The drawing under review shows one solid part. Ordinate dimensions are in mm from its lowest x, y, z. A direction names the side the tool comes from. Coordinates: 2 decimals unless noted, no trailing zeros. Loops run counter-clockwise (first coordinate to the right, second up) from the corner with the lowest first, then second, coordinate; pieces in that order, holes last. Notation, with made-up numbers: M 28,38 L 80,38 A22 cw 80,75 Z; hole C 65.25,41.25 d7. An arc over 180 degrees is marked long. Answer as CSV lines item,"result". Start each with the question number.
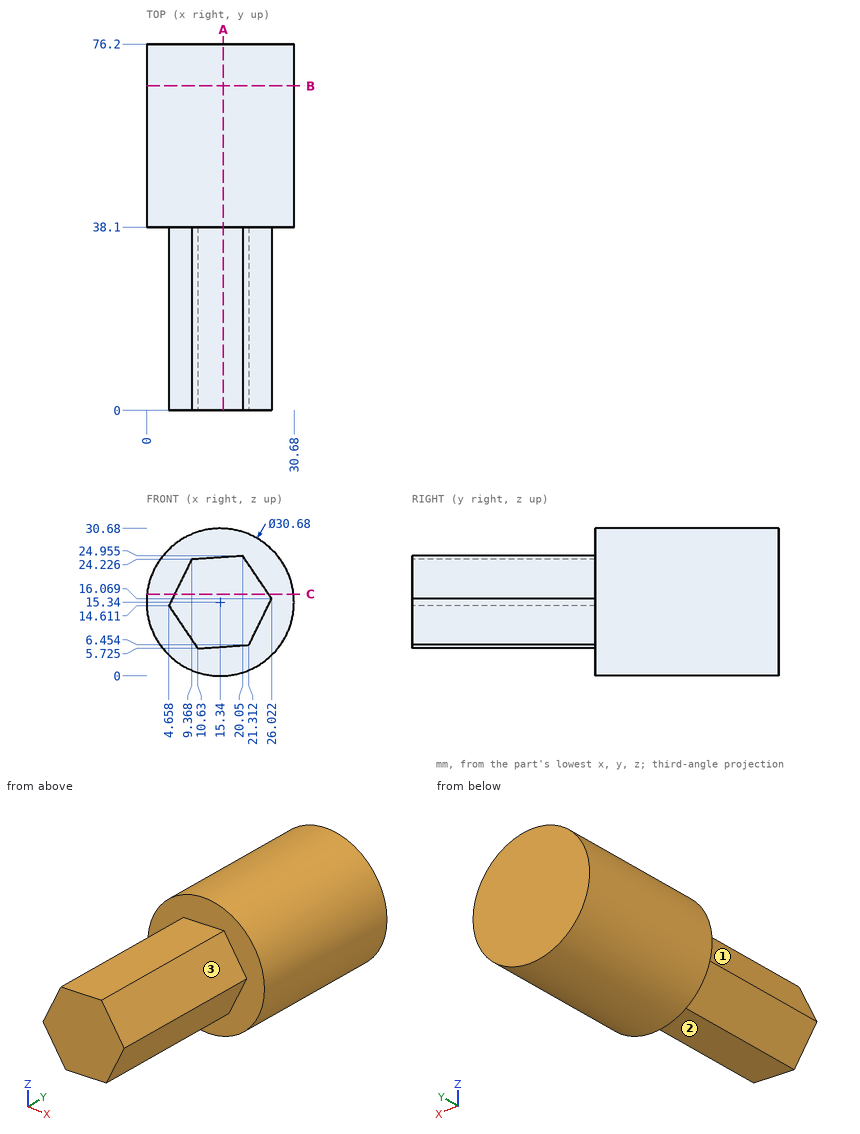
Item 1: For the marked faces 1, 2 and 3, list the 3-axis set-ups (+Z, -Z, +X, -X, +Y, -Y) from which the entire face can be reached by the end or side of a thin tool; tool diameter is ignored.
Item 2: Add section B-B (y = 67.5). Give the boundary of the cut face in (x, z), plus the area to 3 significant figures.
Item 3: For pin 1 (1.5 mm diameter, centred on x = 14.5, y = 61.5, fed in from +Z); pin 2 (8 mm diameter, centred on y = 56.5, z = 26.5, fed in from +X); pin 3 (2 mm diameter, centred on x = 6.5, y = 39.5, fed in from +Z) (1 decimal); pin 4 (2 mm diameter, centred on x = 23.5, y = 41, fed in from +Z), all flat-tipped, find the tip position at first contact; note any pin that passes through.
Item 4: For line 1 along Y through (x, z) = (28.5, 10.5); line 2 along Z through (x, y) = (15.5, 52.5); line 3 along Z through (x, y) = (6.5, 33.5) (1 decimal), list the stretches that pass through material, from the lowest coordinate up. Write a range as from..to.
Item 5: Add section A-A (x = 16). Give the boundary of the cut face in (y, z).
Item 6: Add section C-C (z = 17). Give the boundary of the cut face in (x, y).
Response:
1,face 1,"+Z, -X, -Y"
1,face 2,"-Z, +X, -Y"
1,face 3,"+Z, +X, -Y"
2,outline,"C 15.34,15.34 d30.68"
2,area,"739 mm²"
3,pin 1,"z = 30.68"
3,pin 2,"x = 28.91"
3,pin 3,"z = 28.5"
3,pin 4,"z = 28.91"
4,line 1,"38.1..76.2"
4,line 2,"0..30.68"
4,line 3,"11.9..18.4"
5,outline,"M 0,6.09 L 38.1,6.09 L 38.1,0.01 L 76.2,0.01 L 76.2,30.67 L 38.1,30.67 L 38.1,24.68 L 0,24.68 Z"
6,outline,"M 0.09,38.1 L 5.83,38.1 L 5.83,0 L 25.4,0 L 25.4,38.1 L 30.59,38.1 L 30.59,76.2 L 0.09,76.2 Z"
